```python
from build123d import *

# Parameters (mm, degrees)
SKETCH_1_R      = 1.45
SKETCH_1_R_2    = 5.15
EXTRUDE_1_DEPTH = 8
SKETCH_2_R      = 5.305373799
SKETCH_2_R_2    = 1.85
EXTRUDE_2_DEPTH = 4


with BuildPart() as part:
    # Эскиз1 → Бобышка-Вытянуть1 (new body)
    with BuildSketch(Plane.XY):
        with BuildLine():
            Line((0, 7.65), (45, 7.65))
            ThreePointArc((45, 7.65), (52.65, 0), (45, -7.65))
            Line((45, -7.65), (0, -7.65))
            ThreePointArc((0, -7.65), (-7.65, 0), (0, 7.65))
        make_face()
        Circle(SKETCH_1_R, mode=Mode.SUBTRACT)
        with Locations((45, 0)):
            Circle(SKETCH_1_R, mode=Mode.SUBTRACT)
        with Locations((22.5, 0)):
            Circle(SKETCH_1_R_2, mode=Mode.SUBTRACT)
    extrude(amount=EXTRUDE_1_DEPTH)

    # Эскиз2 → Бобышка-Вытянуть2 (add)
    with BuildSketch(Plane(origin=(0, 0, 0), x_dir=(-1, 0, 0), z_dir=(0, 0, -1))):
        with Locations((-22.5, 0)):
            Circle(SKETCH_2_R)
        with Locations((-22.5, 0)):
            Circle(SKETCH_2_R_2, mode=Mode.SUBTRACT)
    extrude(amount=-EXTRUDE_2_DEPTH)


solid = part.part
```
Check sheet for the modelled part. Datum: model origin and axes. Units: mm. A direction names the side the tool comes from. Coordinates: 2 decimals unless noted, no trailing zeros. Order: outer loops, then holes, each group sorted by start corner. A loop starts at its lowest first (then second) coordinate and runs counter-clockwise, first axis right, second up. Notation, with made-up numbers: (-3, 89.5) -> (32, 89.5) arc R29 cw to (32, 114.5) -> close; hole circle Ø2 at (-28.75, -22.75). An arc over 180 degrees is marked (long way). Write item = value, one per line. Start each with the question number.
1) Mould release check, pull along Y, two halves, no side actions. Record for faces 3 (the flat face through (23, -7.65, 4)), 4 (the flat face through (22, 7.65, 4)), 5 (the cylindrical face through (24.35, 0.08, 1.97)): +Y half, -Y half, draft (parallel to the pull), parting line (faces both ways), or undercut.
2) Access from +Z, -Z, +X, -X, +Y, -Y to the whole of each face (thin tool, end or side, straight path). Record for faces 1 (the cylindrical face through (17.355, 0.226, 5.972)), 2 (the flat face through (23, 2, 0)).
3) Cross-section at A-A (y = 0). Enter the section's corners in (x, z), then the cut area to 3 significant figures.
4) Material ranges on L1, parallel to Y at x = 22.5, z = 6.6; L2, parallel to Y at x = 0, z = 1.5; L3, parallel to X at y = 0.75, z = 7.5, recorded low to high.
5) Go/stop test with flat-tipped pins: P1, Ø1, axis at y = -2.5, z = 1, coming from the +X side; P2, Ø6, axis at x = 22.5, y = 0, coming from the +Z side; P3, Ø1.7, axis at x = 45, y = 0, coming from the -Z side. Record where each tip stops, or that it passes through.
6) Cross-section at D-D (y = -3.75). Enter the section's corners in (x, z).
7) Cross-section at B-B (x = 22.5). Enter the section's corners in (y, z), then the cut area to 3 significant figures.
8) Cross-section at C-C (z = 2.25). Enter the section's corners in (x, y), then the cut area to 3 significant figures.
Ans:
q1.face_3 = -Y half
q1.face_4 = +Y half
q1.face_5 = undercut
q2.face_1 = +Z
q2.face_2 = -Z, +X, -X, +Y, -Y
q3.outline = (-7.65, 0) -> (-1.45, 0) -> (-1.45, 8) -> (-7.65, 8) -> close; (1.45, 0) -> (20.65, 0) -> (20.65, 4) -> (17.35, 4) -> (17.35, 8) -> (1.45, 8) -> close; (24.35, 0) -> (43.55, 0) -> (43.55, 8) -> (27.65, 8) -> (27.65, 4) -> (24.35, 4) -> close; (46.45, 0) -> (52.65, 0) -> (52.65, 8) -> (46.45, 8) -> close
q3.area = 380 mm²
q4.L1 = -7.65 to -5.15, 5.15 to 7.65
q4.L2 = -7.65 to -1.45, 1.45 to 7.65
q4.L3 = -7.61 to -1.24, 1.24 to 17.4, 27.6 to 43.76, 46.24 to 52.61
q5.P1 = 52.38
q5.P2 = 4
q5.P3 = through
q6.outline = (-6.67, 0) -> (51.67, 0) -> (51.67, 8) -> (26.03, 8) -> (26.03, 4) -> (18.97, 4) -> (18.97, 8) -> (-6.67, 8) -> close
q7.outline = (-7.65, 0) -> (-1.85, 0) -> (-1.85, 4) -> (-5.15, 4) -> (-5.15, 8) -> (-7.65, 8) -> close; (1.85, 0) -> (7.65, 0) -> (7.65, 8) -> (5.15, 8) -> (5.15, 4) -> (1.85, 4) -> close
q7.area = 66.4 mm²
q8.outline = (0, -7.65) -> (45, -7.65) arc R7.65 ccw to (45, 7.65) -> (0, 7.65) arc R7.65 ccw to start; hole circle Ø2.9 at (0, 0); hole circle Ø3.7 at (22.5, 0); hole circle Ø2.9 at (45, 0)
q8.area = 848 mm²
